Can you work these out from the model? Positions are in its coordinate system, mm. A direction names the side the tool comes from. Coordinates: 2 decimals unless noted, no trailing zeros. Order: outer loops, then holes, each group sorted by start corner. A loop starts at its lowest first (then second) coordinate and runs counter-clockwise, first axis right, second up. Notation, with made-up numbers: (-32, 14.5) -> (-24, 14.5) arc R27 cw to (-24, 52.5) -> close; hole circle Ø7 at (-27, -11.75). An arc over 180 degrees is marked (long way). Return JSON: item names as keys, results as strings. Group by question number.
1) For faces 4 (the cylindrical face through (-44.44, -200.125, 13.745)), 5 (the cylindrical face through (190.764, -60.075, 31.883)), which set-ups out of +Z, -Z, +X, -X, +Y, -Y let a thin tool reach every point of the face, with its end or its side?
2) If we section it at C-C, the plane z = 11: Please give me the cut outline in (x, y).
3) If we section it at A-A, the plane y = 0: Please give me the cut outline in (x, z), then the cut area to 3 significant figures.
4) If I drill on probe 1 along X at (y, z) = (71, 7); probe 2 along X at (y, z) = (-128, 20.5); probe 3 along Z at (x, y) = (30.5, -101.5), over which ranges is the centre line in solid material (lowest first)? Write a range as from..to.
5) For pin 1 (8 mm diameter, centred on y = -36, z = 29.5, fed in from -X); pin 2 (6 mm diameter, centred on x = -128.5, z = 48.5, fed in from -Y); pin 3 (5 mm diameter, centred on y = 100, z = 49, fed in from +X), each with a flat end and sliding along its axis, tell me the tip position at first contact or that it passes through.
6) Thinking about a two-plate mould opening in Z: for faces 1 (the cylindrical face through (-44.44, -200.125, 45.86)), 2 (the flat face through (-3, 3, 0)), 3 (the flat face through (-196, 45, 27.88)), which applies, +Z half, -Z half, draft (parallel to the pull), parting line (faces both ways), or undercut?
from build123d import *

# Parameters (mm, degrees)
ESQUISSE1_R        = 205
BOSS_EXTRU_1_DEPTH = 56
ESQUISSE3_W        = 5
ESQUISSE3_H        = 8.12


with BuildPart() as part:
    # Esquisse1 → Boss.-Extru.1 (new body)
    with BuildSketch(Plane.XY):
        Circle(ESQUISSE1_R)
    extrude(amount=BOSS_EXTRU_1_DEPTH)

    # Esquisse2 → Enlèvement de matière-Révolution6 (revolve, cut)
    with BuildSketch(Plane(origin=(0, 0, 0), x_dir=(1, 0, 0), z_dir=(0, 1, 0))):
        with BuildLine():
            Line((0, -2095.724246069), (0, -45.724246069))
            ThreePointArc((0, -45.724246069), (1449.568901432, -646.155344636), (2050, -2095.724246069))
            Line((2050, -2095.724246069), (0, -2095.724246069))
        make_face()
    revolve(axis=Axis((0, 0, 0), (0, 0, 1)), mode=Mode.SUBTRACT)

    # Esquisse3 → Enlèvement de matière-Révolution7 (revolve, cut)
    with BuildSketch(Plane(origin=(0, 0, 0), x_dir=(1, 0, 0), z_dir=(0, 1, 0))):
        with Locations((202.5, -31.94)):
            Rectangle(ESQUISSE3_W, ESQUISSE3_H)
    revolve(axis=Axis((0, 0, 2095.724246069), (0, 0, -1)), mode=Mode.SUBTRACT)


solid = part.part
Result sheet:
{
 "1": {"face 4": "+Z, -Z", "face 5": "none"},
 "2": {"outline": "circle Ø410 at (0, 0)"},
 "3": {"outline": "(-205, 0) -> (205, 0) -> (205, 27.88) -> (200, 27.88) -> (200, 36) -> (205, 36) -> (205, 56) arc R2050 cw to (-205, 56) -> (-205, 36) -> (-200, 36) -> (-200, 27.88) -> (-205, 27.88) -> close", "area": "20,100 mm2"},
 "4": {"probe 1": "x = -192.31..192.31", "probe 2": "x = -160.13..160.13", "probe 3": "z = 0..48.47"},
 "5": {"pin 1": "stops at x = -202.43", "pin 2": "stops at y = -162.09", "pin 3": "stops at x = 180.33"},
 "6": {"face 1": "draft", "face 2": "-Z half", "face 3": "undercut"}
}
